Source: CAD feature listing. Evaluate the final solid. Frame: model axes, mm. A direction names the side the tool comes from. Round coordinates to 2 decimals unless told otherwise and drop trailing zeros. Write each loop counter-clockwise with the first axis right and the second up, starting at its lowest first coordinate (ties: lowest second). Pieces come first, ordered by that corner, then holes. Notation, with made-up numbers: (7, 89) - (59, 89) arc R21 cw to (59, 122) - close; hole circle Ø3 at (11.25, 10). An arc over 180 degrees is marked (long way). Write item = value, one per line. Start each with the question number.
```python
from build123d import *

# Parameters (mm, degrees)
SKETCH1_R           = 2.5
BOSS_EXTRUDE1_DEPTH = 120
SKETCH2_R           = 4
BOSS_EXTRUDE2_DEPTH = 4
BOSS_EXTRUDE3_START = -20
SKETCH3_R           = 2.5
BOSS_EXTRUDE3_DEPTH = 20


with BuildPart() as part:
    # Sketch1 → Boss-Extrude1 (new body)
    with BuildSketch(Plane(origin=(0, 0, 0), x_dir=(1, 0, 0), z_dir=(0, 1, 0))):
        with Locations(Location((0, 0, 0), (0, 0, 270))):
            Circle(SKETCH1_R)
    extrude(amount=BOSS_EXTRUDE1_DEPTH)

    # Sketch2 → Boss-Extrude2 (add)
    with BuildSketch(Plane(origin=(0, 0, 0), x_dir=(1, 0, 0), z_dir=(0, 1, 0))):
        with Locations(Location((0, 0, 0), (0, 0, 270))):
            Circle(SKETCH2_R)
    extrude(amount=-BOSS_EXTRUDE2_DEPTH)

    # Sketch3 → Boss-Extrude3 (add)
    with BuildSketch(Plane(origin=(0, 0, 0), x_dir=(1, 0, 0), z_dir=(0, 1, 0)).offset(BOSS_EXTRUDE3_START)):
        with Locations(Location((0, 0, 0), (0, 0, 270))):
            Circle(SKETCH3_R)
    extrude(amount=BOSS_EXTRUDE3_DEPTH)


solid = part.part
```
(1) Section A-A (z = 0). Return the cut outline in (x, y), plus the area to 3 significant figures.
(2) Reachability of faces 1 (the flat face through (0, 120, 0)), 2 (the flat face through (2, 0, 2)), 3 (the flat face through (2, -4, 2)) from +Z, -Z, +X, -X, +Y, -Y: full face, straight path, thin tool, end or side. Return the list, or none.
(3) Section B-B (x = 0). Return the cut outline in (y, z).
(4) Contact query for flat-ended pins moving along their axis: P1, Ø1.5, axis at y = 94.5, z = -3, coming from the -X side; P2, Ø1, axis at y = 61, z = 2.5, coming from the -X side. Output: stop coordinate, or through.
(5) Ray query, L1, parallel to Y at x = -2.25, z = 1.75; L2, parallel to X at y = 36.5, z = 0.25; L3, parallel to Z at x = -0.5, y = 66. Return the intervals inside material, ascending. Write a range as from..to.
(6) Section C-C (y = 66). Return the cut outline in (x, z), plus the area to 3 significant figures.
Solution:
q1.outline = (-4, -4) - (-2.5, -4) - (-2.5, -20) - (2.5, -20) - (2.5, -4) - (4, -4) - (4, 0) - (2.5, 0) - (2.5, 120) - (-2.5, 120) - (-2.5, 0) - (-4, 0) - close
q1.area = 712 mm^2
q2.face_1 = +Z, -Z, +X, -X, +Y
q2.face_2 = +Y
q2.face_3 = -Y
q3.outline = (-20, -2.5) - (-4, -2.5) - (-4, -4) - (0, -4) - (0, -2.5) - (120, -2.5) - (120, 2.5) - (0, 2.5) - (0, 4) - (-4, 4) - (-4, 2.5) - (-20, 2.5) - close
q4.P1 = -1.09
q4.P2 = -1.5
q5.L1 = -4..0
q5.L2 = -2.49..2.49
q5.L3 = -2.45..2.45
q6.outline = circle Ø5 at (0, 0)
q6.area = 19.6 mm^2
